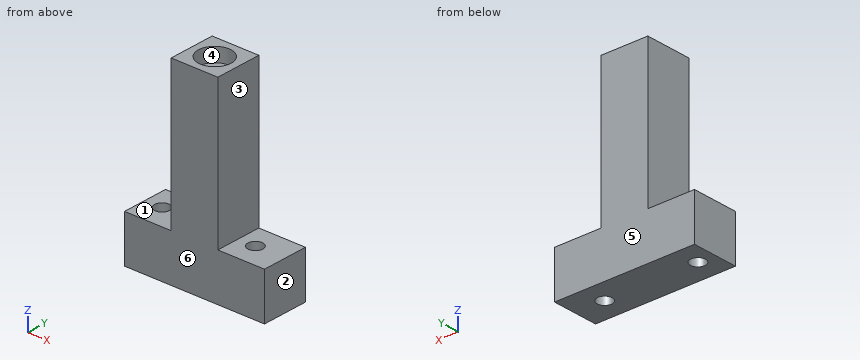
Autodesk Inventor part; units mm, degrees
ref_plane "Work Plane2" through (-21.0916, 0, 41.5167) normal (0, 0, -1) x (0, 1, 0)
ref_plane "YZ Plane" through (0, 0, 0) normal (1, 0, 0) x (0, 1, 0)
ref_plane "XZ Plane" through (0, 0, 0) normal (0, 1, 0) x (-1, 0, 0)
ref_plane "Work Plane1" through (0, 0, 0) normal (0, 0, 1) x (1, 0, 0)
sketch "Sketch1" plane through (0, 0, 0) normal (0, 0, 1) x (1, 0, 0)
  circle A0 centre (45.9084, 5) radius 1.45
  circle A1 centre (25.9084, 5) radius 1.45
  line L0 (-21.0053, 0) -> (95.5084, 0)
  line L1 (95.5084, 10) -> (-17.0053, 10)
  line L2 (22.2515, 0) -> (52.2515, 0)
  line L3 (52.2515, 0) -> (52.2515, 10)
  line L4 (52.2515, 10) -> (22.2515, 10)
  line L5 (22.2515, 10) -> (22.2515, 0)
  line L6 (22.2515, 0) -> (52.2515, 10) construction
  line L7 (52.2515, 0) -> (22.2515, 10) construction
  circle A2 centre (45.9084, 5) radius 1.6
  circle A3 centre (25.9084, 5) radius 1.6
  point P0 (0, 0)
  point P1 (37.2515, 5)
  dimension "d0" = 30
  dimension "d1" = 3.2
  dimension "d2" = 3.2
extrude "Extrusion1" add sketch "Sketch1" along normal blind 10 contours L5 L1 L3 L0
sketch "Sketch2" plane through (0, 0, 10) normal (0, 0, 1) x (1, 0, 0)
  line L0 (95.5084, 10) -> (-17.0053, 10)
  circle A0 centre (-15.5458, 215.5) radius 2.15
  circle A1 centre (-15.5458, 5) radius 2.15
  circle A2 centre (88.9625, 5) radius 2.15
  circle A3 centre (88.9625, 215.5) radius 2.15
  circle A4 centre (-6.0916, 148.2) radius 1.45
  circle A5 centre (77.9084, 141.8) radius 1.45
  circle A6 centre (71.5084, 15.8) radius 1.45
  circle A7 centre (-6.0916, 15.8) radius 1.45
  circle A8 centre (-12.2916, 22) radius 1.45
  circle A9 centre (77.7084, 22) radius 1.45
  circle A10 centre (71.5084, 148.2) radius 1.45
  circle A11 centre (-12.2916, 143.3875) radius 1.45
  arc A12 (-3.9916, 144.2) -> (-7.9916, 140.2) centre (-3.9916, 140.2) ccw
  line L1 (-3.9916, 144.2) -> (69.4084, 144.2)
  arc A13 (73.4084, 140.2) -> (69.4084, 144.2) centre (69.4084, 140.2) ccw
  line L2 (73.4084, 140.2) -> (73.4084, 24.1)
  arc A14 (69.4084, 20.1) -> (73.4084, 24.1) centre (69.4084, 24.1) ccw
  line L3 (69.4084, 20.1) -> (-3.9916, 20.1)
  arc A15 (-7.9916, 24.1) -> (-3.9916, 20.1) centre (-3.9916, 24.1) ccw
  line L4 (-7.9916, 24.1) -> (-7.9916, 140.2)
  line L5 (-21.0053, 220.5) -> (-21.0053, 0)
  line L6 (-21.0053, 0) -> (95.5084, 0)
  line L7 (95.5084, 0) -> (95.5084, 220.5)
  line L8 (95.5084, 220.5) -> (-21.0053, 220.5)
  line L9 (52.2515, 0) -> (52.2515, 10)
  line L10 (22.2515, 10) -> (22.2515, 0)
  line L11 (-21.0053, 0) -> (95.5084, 0)
  line L12 (42.2515, 10) -> (32.2515, 10)
  line L13 (32.2515, 10) -> (32.2515, 0)
  line L14 (32.2515, 0) -> (42.2515, 0)
  line L15 (42.2515, 0) -> (42.2515, 10)
  line L16 (42.2515, 10) -> (32.2515, 0) construction
  line L17 (32.2515, 10) -> (42.2515, 0) construction
  point P0 (0, 0)
  point P1 (37.2515, 5)
  dimension "d5" = 10
  dimension "d6" = 10
ref_plane "Work Plane2" through (-21.0916, 0, 41.5167) normal (0, 0, -1) x (0, 1, 0)
extrude "Extrusion2" add sketch "Sketch2" along normal up to surface (31.5167 mm away) contours L15 L6 L13 L0
sketch "Sketch3" plane through (32.2515, 10, 41.5167) normal (0, 0, 1) x (1, 0, 0)
  line L0 (10, -10) -> (10, 0)
  line L1 (0, 0) -> (0, -10)
  line L2 (-49.2569, 0) -> (63.2569, 0)
  line L3 (63.2569, -10) -> (-53.3431, -10)
  circle A0 centre (-47.7973, -5) radius 3.5
  circle A1 centre (4.9569, -5) radius 3.5
  point P0 (-32.2515, -10)
hole "Hole1" at (37.2084, 5, 41.5167) direction (0, 0, -1) diameter 2.9 depth 25 tip angle 118 counterbore diameter 7 counterbore depth 3
properties part number "00_3rdleg"
The listing builds one solid part. Answer for the finished solid, in the listing's coordinates (mm). Face numbers are marked on the shaded views. A direction names the side the tool comes from. Round coordinates to 2 decimals unless told otherwise and drop trailing zeros. Order: outer loops, then holes, each group sorted by start corner. A loop starts at its lowest first (then second) coordinate and runs counter-clockwise, first axis right, second up. Notation, with made-up numbers: (-5, -25.75) -> (1, -25.75) arc R20 cw to (1, -20.75) -> close; hole circle Ø5 at (23, -28.75). An arc over 180 degrees is marked (long way). Write each question's results on one line, items separated by ' | '. Start each with the question number.
Q1. Find section D-D (z = 14). Determine the outline of the cut face in (x, y).
Q2. Straight lines are drawn through the part: probe 1 along X at (y, z) = (5, 39.75); probe 2 along Z at (x, y) = (28.5, 8); probe 3 along X at (y, z) = (8.25, 31.5). For each, find the intervals that lie inside material, in ascending order. Write a range as from..to.
Q3. Each of these flat-tipped pins is pushed along its axis until it touches: pin 1 (1 mm diameter, centred on x = 46, y = 8, fed in from +Z); pin 2 (5 mm diameter, centred on y = 3.5, z = 30, fed in from -X); pin 3 (4.5 mm diameter, centred on x = 37.21, y = 5, fed in from +Z). Where does it stop, or does it pass through?
Q4. Find section B-B (y = 1). Determine the outline of the cut face in (x, z), then the cut area to 3 significant figures.
Q5. The mould has two halves that part along Y. Classify the marked faces 4, 5 and 6: pulls with the +Y half, pulls with the -Y half, needs draft (parallel to the pull), parting line crosses it, or undercut.
Q6. Find section C-C (x = 35). Determine the outline of the cut face in (y, z).
Q7. Which of the six approach directions +Z, -Z, +X, -X, +Y, -Y give full straight-line access (tool end or side, diameter ignored) to the marked faces 1, 2 and 3?
Q8. Find section A-A (z = 8). Determine the outline of the cut face in (x, y).
Worked answers:
1) outline: (32.25, 0) -> (42.25, 0) -> (42.25, 10) -> (32.25, 10) -> close
2) probe 1: x = 32.25..33.71, 40.71..42.25 | probe 2: z = 0..10 | probe 3: x = 32.25..42.25
3) pin 1: stops at z = 10 | pin 2: stops at x = 32.25 | pin 3: stops at z = 38.52
4) outline: (22.25, 0) -> (52.25, 0) -> (52.25, 10) -> (42.25, 10) -> (42.25, 41.52) -> (32.25, 41.52) -> (32.25, 10) -> (22.25, 10) -> close | area: 615 mm2
5) face 4: undercut | face 5: pulls with the +Y half | face 6: pulls with the -Y half
6) outline: (0, 0) -> (10, 0) -> (10, 41.52) -> (7.72, 41.52) -> (7.72, 38.52) -> (2.28, 38.52) -> (2.28, 41.52) -> (0, 41.52) -> close
7) face 1: +Z, -X, +Y, -Y | face 2: +Z, -Z, +X, +Y, -Y | face 3: +Z, +X, +Y, -Y
8) outline: (22.25, 0) -> (52.25, 0) -> (52.25, 10) -> (22.25, 10) -> close; hole circle Ø3.2 at (25.91, 5); hole circle Ø3.2 at (45.91, 5)
